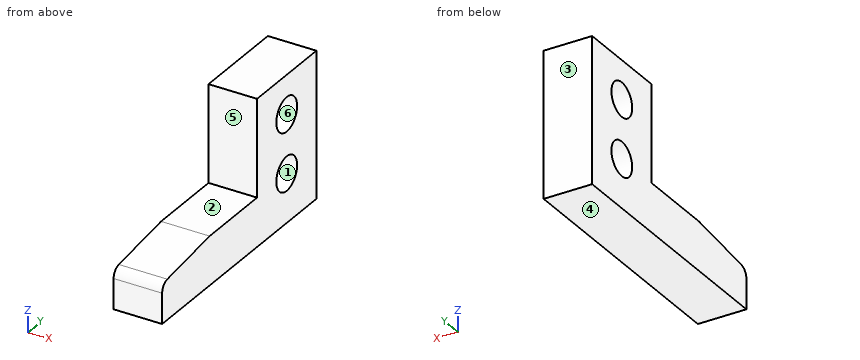
```python
from build123d import *

# Parameters (mm, degrees)
F0_R     = 1.75
F1_DEPTH = 5
F2_SIZE2 = 8
F2_SIZE  = 1
F3_R     = 1


with BuildPart() as f1:
    # F0 (on Right) → F1 (new body)
    with BuildSketch(Plane.YZ):
        Polygon((0, 5), (0, 0), (26, 0), (26, 15), (16, 15), (16, 5), align=None)
        with Locations((21, 5)):
            Circle(F0_R, mode=Mode.SUBTRACT)
        with Locations((21, 11)):
            Circle(F0_R, mode=Mode.SUBTRACT)
    extrude(amount=F1_DEPTH)

    # F2
    f2_edges = [f1.edges().sort_by_distance(p)[0] for p in [
        (2.5, 0, 5),
    ]]
    f2_side = f1.faces().sort_by_distance((2.5, 0, 2.5))[0]
    chamfer(f2_edges, length=F2_SIZE, length2=F2_SIZE2, reference=f2_side)

    # F3
    f3_edges = [f1.edges().sort_by_distance(p)[0] for p in [
        (2.5, 0, 4),
    ]]
    fillet(f3_edges, radius=F3_R)


solid = f1.part
```
Verification items for the finished model (mm, model axes). Face numbers are marked on the shaded views. A direction names the side the tool comes from. Coordinates: 2 decimals unless noted, no trailing zeros. Write each loop counter-clockwise with the first axis right and the second up, starting at its lowest first coordinate (ties: lowest second). Pieces come first, ordered by that corner, then holes. Notation, with made-up numbers: M -31.5,68.5 L 22.5,68.5 A13 ccw 22.5,88.5 Z; hole C -32.75,10.5 d11. An arc over 180 degrees is marked long. One line per item, written item: value.
Item 1: Section check B-B, the plane x = 4.15. Record the boundary of the cut face in (y, z), plus the area to 3 significant figures.
Check sheet entries:
outline: M 0,0 L 26,0 L 26,15 L 16,15 L 16,5 L 8,5 L 0.88,4.11 A1 ccw 0,3.12 Z; hole C 21,5 d3.5; hole C 21,11 d3.5
area: 207 mm^2
Item 2: Access from +Z, -Z, +X, -X, +Y, -Y to the whole of each face (thin tool, end or side, straight path). Record for the marked faces 1 and 2.
Check sheet entries:
face 1: +X, -X
face 2: +Z, +X, -X, -Y
Item 3: Gauge pin test, flat ends, axial feed: pin 1 Ø2 at (y, z) = (17.5, 6) entering from -X; pin 2 Ø2 at (y, z) = (21, 11) entering from -X; pin 3 Ø3 at (x, y) = (3, 6.5) entering from +Z. Record the tip position at first contact, or that the pin passes through.
Check sheet entries:
pin 1: stops at x = 0
pin 2: passes through
pin 3: stops at z = 5
Item 4: Section check D-D, the plane z = 9. Record the boundary of the cut face in (x, y).
Check sheet entries:
outline: M 0,16 L 5,16 L 5,26 L 0,26 Z
Item 5: Section check C-C, the plane z = 11. Record the boundary of the cut face in (x, y), plus the area to 3 significant figures.
Check sheet entries:
outline: M 0,16 L 5,16 L 5,19.25 L 0,19.25 Z; M 0,22.75 L 5,22.75 L 5,26 L 0,26 Z
area: 32.5 mm^2
Item 6: Scan lines: line 1 along Z through (x, y) = (1.15, 21); line 2 along Y through (x, z) = (1, 8); line 3 along Y through (x, z) = (2.1, 10.5). Record each from-to range of solid material in increasing order.
Check sheet entries:
line 1: z = 0 to 3.25, 6.75 to 9.25, 12.75 to 15
line 2: y = 16 to 26
line 3: y = 16 to 19.32, 22.68 to 26
Item 7: Section check A-A, the plane y = 21. Record the boundary of the cut face in (x, z).
Check sheet entries:
outline: M 0,0 L 5,0 L 5,3.25 L 0,3.25 Z; M 0,6.75 L 5,6.75 L 5,9.25 L 0,9.25 Z; M 0,12.75 L 5,12.75 L 5,15 L 0,15 Z
Item 8: Mould release check, pull along Y, two halves, no side actions. Record for the marked faces 3, 4, 5 and 6: pulls with the +Y half, pulls with the -Y half, needs draft (parallel to the pull), parting line crosses it, or undercut.
Check sheet entries:
face 3: pulls with the +Y half
face 4: needs draft
face 5: pulls with the -Y half
face 6: undercut
